```python
from build123d import *

# Parameters (mm, degrees)
BOSS_EXTRUDE1_DEPTH  = 3
SKETCH2_W            = 15
SKETCH2_H            = 12
CUT_EXTRUDE1_DEPTH   = 68.948509917
FILLET1_R            = 1
CUT_EXTRUDE2_DEPTH   = 68.948509917
LPATTERN1_COUNT      = 4
LPATTERN1_PITCH      = 10
LPATTERN1_COUNT_DIR2 = 4
LPATTERN1_PITCH_DIR2 = 6


with BuildPart() as part:
    # Sketch1 → Boss-Extrude1 (new body)
    with BuildSketch(Plane.XY):
        Polygon((0, 0), (0, 45), (12.5, 45), (12.5, 48), (32.5, 48), (32.5, 45), (48, 45), (48, 27.5), (45, 27.5), (45, 17.5), (48, 17.5), (48, 0), (32.5, 0), (32.5, -6), (12.5, -6), (12.5, 0), align=None)
    extrude(amount=BOSS_EXTRUDE1_DEPTH)

    # Sketch2 → Cut-Extrude1 (cut, through all)
    with BuildSketch(Plane.XY.offset(3)):
        with Locations((32.5, 11)):
            Rectangle(SKETCH2_W, SKETCH2_H)
    extrude(amount=-CUT_EXTRUDE1_DEPTH, mode=Mode.SUBTRACT)

    # Fillet1
    fillet1_edges = [part.edges().sort_by_distance(p)[0] for p in [
        (25, 5, 1.5),
        (25, 17, 1.5),
        (40, 17, 1.5),
        (40, 5, 1.5),
    ]]
    fillet(fillet1_edges, radius=FILLET1_R)

    # Sketch3 → Cut-Extrude2 (cut, through all)
    with BuildSketch(Plane.XY.offset(3)):
        with BuildLine():
            Line((4, 42), (9, 42))
            ThreePointArc((9, 42), (9.707106781, 41.707106781), (10, 41))
            Line((10, 41), (10, 39))
            ThreePointArc((10, 39), (9.707106781, 38.292893219), (9, 38))
            Line((9, 38), (4, 38))
            ThreePointArc((4, 38), (3.292893219, 38.292893219), (3, 39))
            Line((3, 39), (3, 41))
            ThreePointArc((3, 41), (3.292893219, 41.707106781), (4, 42))
        make_face()
    cut_extrude2 = extrude(amount=-CUT_EXTRUDE2_DEPTH, mode=Mode.SUBTRACT)

    # LPattern1: Cut-Extrude2 4 × 4
    with Locations(*[(i * LPATTERN1_PITCH, -j * LPATTERN1_PITCH_DIR2, 0) for i in range(LPATTERN1_COUNT) for j in range(LPATTERN1_COUNT_DIR2) if (i, j) != (0, 0)]):
        add(cut_extrude2, mode=Mode.SUBTRACT)


solid = part.part
```
Design review of the part built by this model. Coordinates are the model's own, in mm. A direction names the side the tool comes from. Coordinates: 2 decimals unless noted, no trailing zeros. Write each loop counter-clockwise with the first axis right and the second up, starting at its lowest first coordinate (ties: lowest second). Pieces come first, ordered by that corner, then holes. Notation, with made-up numbers: M 37,-10 L 56,-10 A15 cw 56,13 Z; hole C 70.5,8 d3. An arc over 180 degrees is marked long. Answer as a JSON object with one key per item and string values.
Item 1: Add section C-C, the plane y = 11. Give the boundary of the cut face in (x, z).
Outcome:
{"outline": "M 0,0 L 25,0 L 25,3 L 0,3 Z; M 40,0 L 48,0 L 48,3 L 40,3 Z"}
Item 2: Add section B-B, the plane x = 16.5. Give the boundary of the cut face in (y, z), and give its area (3 significant figures).
Outcome:
{"outline": "M -6,0 L 20,0 L 20,3 L -6,3 Z; M 24,0 L 26,0 L 26,3 L 24,3 Z; M 30,0 L 32,0 L 32,3 L 30,3 Z; M 36,0 L 38,0 L 38,3 L 36,3 Z; M 42,0 L 48,0 L 48,3 L 42,3 Z", "area": "114 mm²"}
Item 3: Add section A-A, the plane x = 37. Give the boundary of the cut face in (y, z), and give its area (3 significant figures).
Outcome:
{"outline": "M 0,0 L 5,0 L 5,3 L 0,3 Z; M 17,0 L 20,0 L 20,3 L 17,3 Z; M 24,0 L 26,0 L 26,3 L 24,3 Z; M 30,0 L 32,0 L 32,3 L 30,3 Z; M 36,0 L 38,0 L 38,3 L 36,3 Z; M 42,0 L 45,0 L 45,3 L 42,3 Z", "area": "51.0 mm²"}
Item 4: Draft analysis for pull direction X (two halves, no side actions). For faces 1 (the flat face through (32.5, 47, 1)), 2 (the flat face through (47, 27.5, 1)), 3 (the flat face through (27, 32, 2)), state which applies: pulls with the +X half, pulls with the -X half, needs draft (parallel to the pull), parting line crosses it, or undercut.
Outcome:
{"face 1": "pulls with the +X half", "face 2": "needs draft", "face 3": "undercut"}
Item 5: Add section D-D, the plane x = 5.5. Give the boundary of the cut face in (y, z), and give its area (3 significant figures).
Outcome:
{"outline": "M 0,0 L 20,0 L 20,3 L 0,3 Z; M 24,0 L 26,0 L 26,3 L 24,3 Z; M 30,0 L 32,0 L 32,3 L 30,3 Z; M 36,0 L 38,0 L 38,3 L 36,3 Z; M 42,0 L 45,0 L 45,3 L 42,3 Z", "area": "87.0 mm²"}
Item 6: Wall thickness on probe 1 along Y at (x, z) = (8.5, 0.2); probe 2 along X at (y, z) = (28.5, 2.7); probe 3 along X at (y, z) = (22.5, 2.2): over which ranges is each line inside the solid? List them lowest first.
Outcome:
{"probe 1": "0 to 20, 24 to 26, 30 to 32, 36 to 38, 42 to 45", "probe 2": "0 to 3, 10 to 13, 20 to 23, 30 to 33, 40 to 48", "probe 3": "0 to 3, 10 to 13, 20 to 23, 30 to 33, 40 to 45"}
Item 7: Insertion check: pin 1 Ø0.9 at (x, z) = (6, 1.5) entering from -Y. The pin has a flat end and moves straight along its axis. Give the tip position at first contact, or say it passes through.
Outcome:
{"pin 1": "y = 0"}
Item 8: Machinability: for faces 4 (the flat face through (45, 23, 1)), 5 (the flat face through (23, 40, 2)), 6 (the flat face through (23, -6, 1)), which of the approach directions +Z, -Z, +X, -X, +Y, -Y give a long, thin tool a straight path to every point of the face, cutting with its end or side? Answer none if there is none.
Outcome:
{"face 4": "+Z, -Z, +X", "face 5": "+Z, -Z", "face 6": "+Z, -Z, +X, -X, -Y"}
